Part print with two shaded views. Sizes in mm from the minimum x, y, z corner. Give positions to 0.01 mm unless a question says otherwise; leave off trailing zeros. Loops run counter-clockwise (first coordinate to the right, second up) from the corner with the lowest first, then second, coordinate; pieces in that order, holes last. Notation, with made-up numbers: M 37,-32 L 79,-32 A29 cw 79,6 Z; hole C -37,70 d8. An arc over 180 degrees is marked long. Answer as a JSON object with one key per item and string values. Group by question number.
1. Drill centre lines: line 1 along Z through (x, y) = (7.5, 4.5); line 2 along Z through (x, y) = (4.75, 0.75); line 3 along X through (y, z) = (5.5, 17.5). Where is each one in solid material? Low to high. Write a range as [from, to].
2. Slice it at C-C (y = 5.25). List the corners of the cut face in (x, z).
3. Slice it at B-B (x = 7.5). List the corners of the cut face in (y, z).
4. Slice it at D-D (x = 3). List the corners of the cut face in (y, z).
5. Drop flat-ended pins along their axis: pin 1 Ø4 at (x, y) = (3.5, 6.5) entering from -Z; pin 2 Ø1 at (x, y) = (12, 6.5) entering from +Z. Give the stop position or say it passes through.
6. Slice it at A-A (z = 9.75). List the corners of the cut face in (x, y).
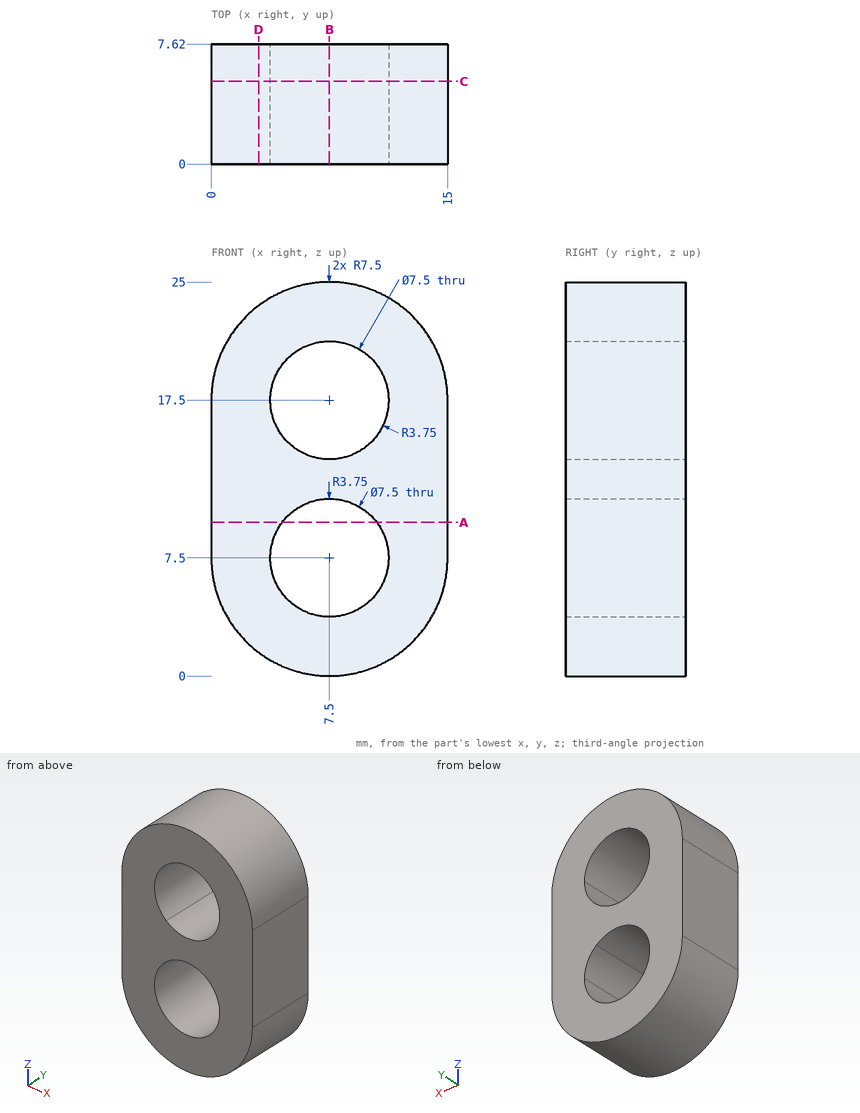
Established:
{
 "1": {"line 1": "z = [0, 3.75], [11.25, 13.75], [21.25, 25]", "line 2": "z = [0.52, 4.95], [10.05, 14.95], [20.05, 24.48]", "line 3": "x = [0, 3.75], [11.25, 15]"},
 "2": {"outline": "M 0,7.5 A7.5 ccw 15,7.5 L 15,17.5 A7.5 ccw 0,17.5 Z; hole M 9.89,10.39 A3.75 ccw long 11.25,7.5 A3.75 ccw Z; hole M 9.89,14.61 A3.75 ccw 11.25,17.5 A3.75 ccw long Z"},
 "3": {"outline": "M 0,0 L 7.62,0 L 7.62,3.75 L 0,3.75 Z; M 0,11.25 L 7.62,11.25 L 7.62,13.75 L 0,13.75 Z; M 0,21.25 L 7.62,21.25 L 7.62,25 L 0,25 Z"},
 "4": {"outline": "M 0,1.5 L 7.62,1.5 L 7.62,23.5 L 0,23.5 Z"},
 "5": {"pin 1": "stops at z = 0.27", "pin 2": "stops at z = 23.84"},
 "6": {"outline": "M 0,0 L 4.5,0 L 4.5,7.62 L 0,7.62 Z; M 10.5,0 L 15,0 L 15,7.62 L 10.5,7.62 Z"}
}
